The listing builds one solid part. Answer for the finished solid, in the listing's coordinates (mm). Coordinates: 2 decimals unless noted, no trailing zeros. Order: outer loops, then holes, each group sorted by start corner. A loop starts at its lowest first (then second) coordinate and runs counter-clockwise, first axis right, second up. Notation, with made-up numbers: (49.5, -21) -> (67.5, -21) arc R19 ccw to (67.5, 15) -> close; hole circle Ø2 at (29.25, -4). An arc over 180 degrees is marked (long way). Return JSON: item names as keys, results as strings.
from build123d import *

# Parameters (mm, degrees)
SKETCH_2_W           = 150
SKETCH_2_H           = 43.5
SKETCH_2_R           = 7.5
SKETCH_2_R_2         = 4.05
EXTRUDE_1_DEPTH      = 8
CUT_EXTRUDE_2_DEPTH  = 157.38494173
SKETCH_5_R           = 1.55
CUT_EXTRUDE_3_DEPTH  = 157.38494173
SKETCH_20_R          = 5.5
CUT_EXTRUDE_17_DEPTH = 157.38494173
CUT_EXTRUDE_5_DEPTH  = 4.5
SKETCH_25_R          = 1.55
CUT_EXTRUDE_13_DEPTH = 157.38494173
CUT_EXTRUDE_11_DEPTH = 2
EXTRUDE_2_DEPTH      = 8


with BuildPart() as part:
    # 草图2 → 凸台-拉伸1 (new body)
    with BuildSketch(Plane.XY):
        with Locations((75, 21.75)):
            Rectangle(SKETCH_2_W, SKETCH_2_H)
        with Locations((10, 8.5)):
            Circle(SKETCH_2_R, mode=Mode.SUBTRACT)
        with Locations((75, 10.5)):
            Circle(SKETCH_2_R_2, mode=Mode.SUBTRACT)
        with Locations((140, 8.5)):
            Circle(SKETCH_2_R, mode=Mode.SUBTRACT)
    extrude_1 = extrude(amount=EXTRUDE_1_DEPTH)

    # 草图4 → 切除-拉伸2 (cut, through all)
    with BuildSketch(Plane(origin=(150, 0, 0), x_dir=(0, 0, -1), z_dir=(1, 0, 0))):
        Polygon((-1.5, 41.7), (-2.5, 41.7), (-2.5, 43.5), (0, 43.5), (0, 38.3), (-1.5, 38.3), align=None)
    cut_extrude_2 = extrude(amount=-CUT_EXTRUDE_2_DEPTH, mode=Mode.SUBTRACT)

    # 草图5 → 切除-拉伸3 (cut, through all)
    with BuildSketch(Plane.XY.offset(8)):
        with Locations((83, 10.5)):
            Circle(SKETCH_5_R)
        with Locations((67, 10.5)):
            Circle(SKETCH_5_R)
    cut_extrude_3 = extrude(amount=-CUT_EXTRUDE_3_DEPTH, mode=Mode.SUBTRACT)

    # 草图20 → 切除-拉伸17 (cut, through all)
    with BuildSketch(Plane(origin=(0, 0, 0), x_dir=(-1, 0, 0), z_dir=(0, 0, -1))):
        with Locations((-75, 10.5)):
            Circle(SKETCH_20_R)
    cut_extrude_17 = extrude(amount=-CUT_EXTRUDE_17_DEPTH, mode=Mode.SUBTRACT)

    # 草图8 → 切除-拉伸5 (cut)
    with BuildSketch(Plane(origin=(0, 0, 0), x_dir=(-1, 0, 0), z_dir=(0, 0, -1))):
        Polygon((-80.15, 8.854551733), (-80.15, 12.145448267), (-83, 13.790896534), (-85.85, 12.145448267), (-85.85, 8.854551733), (-83, 7.209103466), align=None)
        Polygon((-64.15, 8.854551733), (-64.15, 12.145448267), (-67, 13.790896534), (-69.85, 12.145448267), (-69.85, 8.854551733), (-67, 7.209103466), align=None)
    cut_extrude_5 = extrude(amount=-CUT_EXTRUDE_5_DEPTH, mode=Mode.SUBTRACT)

    # 草图25 → 切除-拉伸13 (cut, through all)
    with BuildSketch(Plane(origin=(0, 0, 0), x_dir=(-1, 0, 0), z_dir=(0, 0, -1))):
        with Locations((-130, 34.5)):
            Circle(SKETCH_25_R)
        with Locations((-20, 34.5)):
            Circle(SKETCH_25_R)
    cut_extrude_13 = extrude(amount=-CUT_EXTRUDE_13_DEPTH, mode=Mode.SUBTRACT)

    # 草图19 → 切除-拉伸11 (cut)
    with BuildSketch(Plane(origin=(0, 0, 2.5), x_dir=(-1, 0, 0), z_dir=(0, 0, -1))):
        with BuildLine():
            Line((-60, 43.5), (-90.247938178, 43.5))
            Line((-90.247938178, 43.5), (-90.247938178, 42.7))
            ThreePointArc((-90.247938178, 42.7), (-89.747938178, 42.2), (-89.247938178, 42.7))
            Line((-89.247938178, 42.7), (-61, 42.7))
            ThreePointArc((-61, 42.7), (-60.5, 42.2), (-60, 42.7))
            Line((-60, 42.7), (-60, 43.5))
        make_face()
    cut_extrude_11 = extrude(amount=-CUT_EXTRUDE_11_DEPTH, mode=Mode.SUBTRACT)

    # 草图22 → 凸台-拉伸2 (add)
    with BuildSketch(Plane.XY.offset(8)):
        with BuildLine():
            Line((0, -3), (4.5, -3))
            ThreePointArc((4.5, -3), (3, -1.5), (4.5, 0))
            Line((4.5, 0), (0, 0))
            ThreePointArc((0, 0), (1.5, -1.5), (0, -3))
        make_face()
        with BuildLine():
            Line((150, 0), (145.5, 0))
            ThreePointArc((145.5, 0), (147, -1.5), (145.5, -3))
            Line((145.5, -3), (150, -3))
            ThreePointArc((150, -3), (148.5, -1.5), (150, 0))
        make_face()
    extrude(amount=-EXTRUDE_2_DEPTH)

    # 镜向2: 凸台-拉伸1, 切除-拉伸2, 切除-拉伸3, 切除-拉伸17, 切除-拉伸5, 切除-拉伸13, 切除-拉伸11 across plane
    add(extrude_1.mirror(Plane(origin=(0, -1.5, 0), x_dir=(0, 0, 1), z_dir=(0, -1, 0))))
    add(cut_extrude_2.mirror(Plane(origin=(0, -1.5, 0), x_dir=(0, 0, 1), z_dir=(0, -1, 0))), mode=Mode.SUBTRACT)
    add(cut_extrude_3.mirror(Plane(origin=(0, -1.5, 0), x_dir=(0, 0, 1), z_dir=(0, -1, 0))), mode=Mode.SUBTRACT)
    add(cut_extrude_17.mirror(Plane(origin=(0, -1.5, 0), x_dir=(0, 0, 1), z_dir=(0, -1, 0))), mode=Mode.SUBTRACT)
    add(cut_extrude_5.mirror(Plane(origin=(0, -1.5, 0), x_dir=(0, 0, 1), z_dir=(0, -1, 0))), mode=Mode.SUBTRACT)
    add(cut_extrude_13.mirror(Plane(origin=(0, -1.5, 0), x_dir=(0, 0, 1), z_dir=(0, -1, 0))), mode=Mode.SUBTRACT)
    add(cut_extrude_11.mirror(Plane(origin=(0, -1.5, 0), x_dir=(0, 0, 1), z_dir=(0, -1, 0))), mode=Mode.SUBTRACT)


solid = part.part
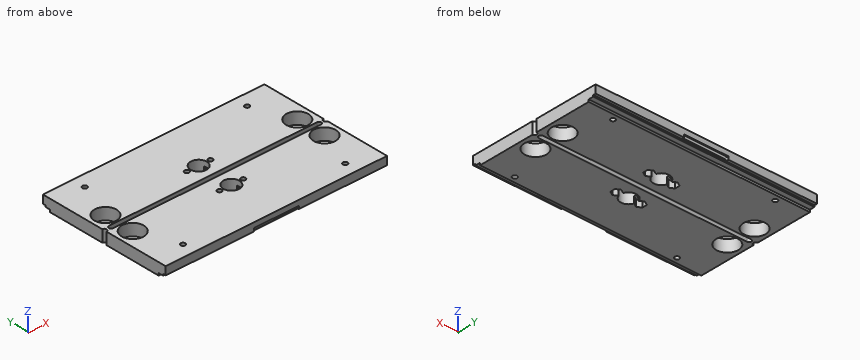
1. The part is cut by section C-C on x = 130. Give the vertices of the cut face in (y, z), and give its area (3 significant figures).
Answer block:
{"outline": "(-46.5, 2.5) -> (-44.7, 2.5) -> (-44.7, 1.5) -> (-41.3, 1.5) -> (-41.3, 0) -> (-39.05, 0) -> (-39.05, 8) -> (-46.5, 8) -> close; (-35.95, 0) -> (-3, 0) -> (-3, 8) -> (-35.95, 8) -> close; (0, 0) -> (32.95, 0) -> (32.95, 8) -> (0, 8) -> close; (36.05, 0) -> (38.3, 0) -> (38.3, 1.5) -> (41.7, 1.5) -> (41.7, 2.5) -> (43.5, 2.5) -> (43.5, 8) -> (36.05, 8) -> close", "area": "627 mm2"}
2. The part is cut by section D-D on x = 77.5. Give the vertices of the cut face in (y, z).
Answer block:
{"outline": "(-46.5, 4.5) -> (-45.7, 4.5) -> (-45.7, 2.5) -> (-44.7, 2.5) -> (-44.7, 1.5) -> (-41.3, 1.5) -> (-41.3, 0) -> (-18.4, 0) -> (-18.4, 8) -> (-46.5, 8) -> close; (-8.6, 0) -> (-3, 0) -> (-3, 8) -> (-8.6, 8) -> close; (0, 0) -> (5.6, 0) -> (5.6, 8) -> (0, 8) -> close; (15.4, 0) -> (38.3, 0) -> (38.3, 1.5) -> (41.7, 1.5) -> (41.7, 2.5) -> (42.7, 2.5) -> (42.7, 4.5) -> (43.5, 4.5) -> (43.5, 8) -> (15.4, 8) -> close"}
3. Each of these flat-tipped pins is pushed along its axis until it touches: pin 1 Ø0.6 at (x, z) = (81.5, 3.5) entering from +Y; pin 2 Ø9 at (x, y) = (140, 8.5) entering from +Z; pin 3 Ø19.5 at (x, y) = (10, -11.5) entering from -Z; pin 4 Ø0.5 at (x, y) = (50.5, -45.5) entering from -Z. Where does it stop, or does it pass through?
Answer block:
{"pin 1": "stops at y = 42.7", "pin 2": "passes through", "pin 3": "stops at z = 0", "pin 4": "stops at z = 2.5"}
4. Consider line 1 (Y direction, x = 10, z = 5.5); line 2 (X direction, y = -37.5, z = 3); line 3 (Y direction, x = 52, z = 6.5). Determine where each line is inside the solid, lowest interval first. Write a range as from..to.
Answer block:
{"line 1": "y = -46.5..-19, -4..-3, 0..1, 16..43.5", "line 2": "x = 0..18.45, 21.55..128.45, 131.55..150", "line 3": "y = -46.5..-3, 0..43.5"}
5. The part is cut by section B-B on x = 102.5. Give the vertices of the cut face in (y, z).
Answer block:
{"outline": "(-46.5, 2.5) -> (-44.7, 2.5) -> (-44.7, 1.5) -> (-41.3, 1.5) -> (-41.3, 0) -> (-3, 0) -> (-3, 8) -> (-46.5, 8) -> close; (0, 0) -> (38.3, 0) -> (38.3, 1.5) -> (41.7, 1.5) -> (41.7, 2.5) -> (43.5, 2.5) -> (43.5, 8) -> (0, 8) -> close"}
6. The part is cut by section A-A on y = -37.5. Give the vertices of the cut face in (x, z), and give its area (3 significant figures).
Answer block:
{"outline": "(0, 0) -> (18.45, 0) -> (18.45, 8) -> (0, 8) -> close; (21.55, 0) -> (128.45, 0) -> (128.45, 8) -> (21.55, 8) -> close; (131.55, 0) -> (150, 0) -> (150, 8) -> (131.55, 8) -> close", "area": "1,150 mm2"}
